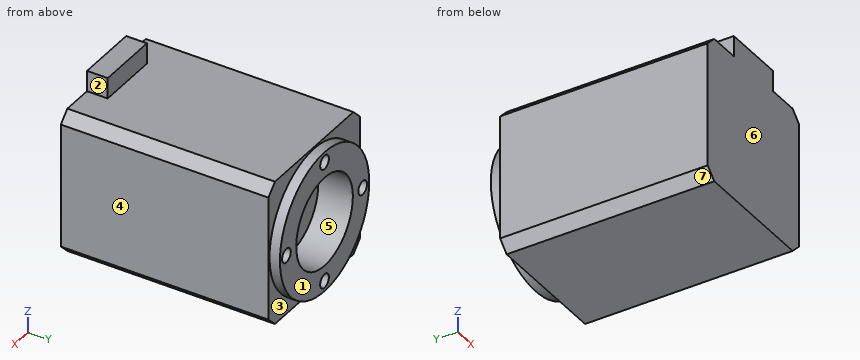
```python
from build123d import *

# Parameters (mm, degrees)
ESQUISSE1_W             = 42
ESQUISSE1_H             = 42
BOSS_EXTRU_1_DEPTH      = 60
ESQUISSE2_R             = 20.5
BOSS_EXTRU_2_DEPTH      = 3
ESQUISSE3_R             = 13
ENL_V_MAT_EXTRU_1_DEPTH = 10
ESQUISSE4_R             = 2
ENL_V_MAT_EXTRU_2_DEPTH = 3.5
CHANFREIN1_SIZE         = 3
ESQUISSE5_W             = 18
ESQUISSE5_H             = 6
BOSS_EXTRU_3_DEPTH      = 6


with BuildPart() as part:
    # Esquisse1 → Boss.-Extru.1 (new body)
    with BuildSketch(Plane(origin=(0, 0, 0), x_dir=(1, 0, 0), z_dir=(0, 1, 0))):
        with Locations((21, 21)):
            Rectangle(ESQUISSE1_W, ESQUISSE1_H)
    extrude(amount=BOSS_EXTRU_1_DEPTH)

    # Esquisse2 → Boss.-Extru.2 (add)
    with BuildSketch(Plane(origin=(0, 60, 0), x_dir=(1, 0, 0), z_dir=(0, 1, 0))):
        with Locations(Location((21, 21, 0), (0, 0, 270))):
            Circle(ESQUISSE2_R)
    extrude(amount=BOSS_EXTRU_2_DEPTH)

    # Esquisse3 → Enlèv. mat.-Extru.1 (cut)
    with BuildSketch(Plane(origin=(0, 63, 0), x_dir=(1, 0, 0), z_dir=(0, 1, 0))):
        with Locations(Location((21, 21, 0), (0, 0, 270))):
            Circle(ESQUISSE3_R)
    extrude(amount=-ENL_V_MAT_EXTRU_1_DEPTH, mode=Mode.SUBTRACT)

    # Esquisse4 → Enlèv. mat.-Extru.2 (cut)
    with BuildSketch(Plane(origin=(0, 63, 0), x_dir=(1, 0, 0), z_dir=(0, 1, 0))):
        with Locations(Location((3.5, 21, 0), (0, 0, 270))):
            Circle(ESQUISSE4_R)
        with Locations(Location((21, 38.5, 0), (0, 0, 270))):
            Circle(ESQUISSE4_R)
        with Locations(Location((38.5, 21, 0), (0, 0, 270))):
            Circle(ESQUISSE4_R)
        with Locations(Location((21, 3.5, 0), (0, 0, 270))):
            Circle(ESQUISSE4_R)
    extrude(amount=-ENL_V_MAT_EXTRU_2_DEPTH, mode=Mode.SUBTRACT)

    # Chanfrein1
    chanfrein1_edges = [part.edges().sort_by_distance(p)[0] for p in [
        (0, 30, -42),
        (42, 30, -42),
        (42, 30, 0),
        (0, 30, 0),
    ]]
    chamfer(chanfrein1_edges, length=CHANFREIN1_SIZE)

    # Esquisse5 → Boss.-Extru.3 (add)
    with BuildSketch(Plane.XY):
        with Locations((21, 3)):
            Rectangle(ESQUISSE5_W, ESQUISSE5_H)
    extrude(amount=BOSS_EXTRU_3_DEPTH)


solid = part.part
```
Geometry: final body of the model. Coordinates: model frame, mm. Face numbers are marked on the shaded views. A direction names the side the tool comes from. Coordinates: 2 decimals unless noted, no trailing zeros. Order: outer loops, then holes, each group sorted by start corner. A loop starts at its lowest first (then second) coordinate and runs counter-clockwise, first axis right, second up.
Item 1: Material intervals for line 1 along X through (y, z) = (60.8, -21); line 2 along Y through (x, z) = (32, -17); line 3 along Z through (x, y) = (15, 39), sorted ascending.
Answer:
line 1: x = 0.5 to 1.5, 5.5 to 8, 34 to 36.5, 40.5 to 41.5
line 2: y = 0 to 53
line 3: z = -42 to 0
Item 2: Draft query along X for the marked faces 4, 5, 6 and 7. Return one class per face: released by +X, released by -X, zero draft, split by the parting line, or undercut.
Answer:
face 4: released by +X
face 5: undercut
face 6: zero draft
face 7: released by -X
Item 3: Section query A-A (y = 58). Output: boundary loops of the cut face in (x, z).
Answer:
outline: (0, -39) - (3, -42) - (39, -42) - (42, -39) - (42, -3) - (39, 0) - (3, 0) - (0, -3) - close; hole circle Ø26 at (21, -21)
Item 4: Section query B-B (y = 15). Output: boundary loops of the cut face in (x, z).
Answer:
outline: (0, -39) - (3, -42) - (39, -42) - (42, -39) - (42, -3) - (39, 0) - (3, 0) - (0, -3) - close
Item 5: Section query D-D (z = 1.5). Output: boundary loops of the cut face in (x, y).
Answer:
outline: (12, 0) - (30, 0) - (30, 6) - (12, 6) - close
Item 6: Contact query for flat-ended pins moving along their axis: P1, Ø4, axis at x = 15, z = -3, coming from the -Y side; P2, Ø3, axis at x = 21, z = -38.5, coming from the +Y side; P3, Ø5, axis at y = 4.5, z = 4, coming from the -X side; P4, Ø1.8, axis at x = 17.5, z = 3, coming from the +Y side. Output: stop coordinate, or through.
Answer:
P1: stops at y = 0
P2: stops at y = 59.5
P3: stops at x = 12
P4: stops at y = 6
Item 7: Section query C-C (x = 24). Output: boundary loops of the cut face in (y, z), then the cut area to 3 significant figures.
Answer:
outline: (0, -42) - (60, -42) - (60, -41.28) - (63, -41.28) - (63, -33.65) - (53, -33.65) - (53, -8.35) - (63, -8.35) - (63, -0.72) - (60, -0.72) - (60, 0) - (6, 0) - (6, 6) - (0, 6) - close
area: 2,420 mm2
Item 8: Access query for the marked faces 1, 2 and 3. Directions: +Z, -Z, +X, -X, +Y, -Y. A direction counts if a zero-diameter tool reaches every point of the face in a straight line with its end or side. Return the directions, or none.
Answer:
face 1: +Z, -Z, +X, -X, +Y
face 2: +Z, +X, +Y, -Y
face 3: +Y
